Here's how the part is built. I have some questions about the finished solid (model axes, mm). A direction names the side the tool comes from. Coordinates: 2 decimals unless noted, no trailing zeros. Write each loop counter-clockwise with the first axis right and the second up, starting at its lowest first coordinate (ties: lowest second). Pieces come first, ordered by that corner, then holes. Notation, with made-up numbers: (-3.75, -27) -> (11.25, -27) arc R20 cw to (11.25, -20) -> close; hole circle Ø7 at (27.5, 74.25). An arc over 180 degrees is marked (long way). Put each result on its own line as item: value. Start each with the question number.
Item 1: On a 3-axis mill with a long thin cutter (end or side, diameter ignored), from which of +Z, -Z, +X, -X, +Y, -Y can I reach the whole of each face in a straight line? I mean faces 1 (the face through (54.8, 2, -30)), 2 (the face through (9, 2, -42.5)), 3 (the face through (-56.5, 1.48, -41.07)). Say none if no direction works.
Item 2: I want a section at B-B, the plane z = 9. List the corners of the cut face in (x, y) for me, then the cut area to 3 significant figures.
Item 3: For pin 1 (0.9 mm diameter, centred on y = 1, z = -33, fed in from +X); pin 2 (1.5 mm diameter, centred on x = -41.5, y = 1.5, fed in from -Z), each with a flat end and sliding along its axis, tell me the tip position at first contact or that it passes through.
Item 4: I want a section at C-C, the plane x = -98. List the corners of the cut face in (y, z) for me, then the cut area to 3 significant figures.
Item 5: If we mould it in two halves opening along X, with no side actions, what happens to faces 4 (the face through (-93.982, 1.521, -1.905)), 5 (the face through (-45, 1, -22.5)), 6 (the face through (73.5, 1.52, -21.07))? For each: released by +X, released by -X, zero draft, split by the parting line, or undercut.
Item 6: I want a section at A-A, the plane y = 0.5. List the corners of the cut face in (x, z) for me, then the cut area to 3 significant figures.
Item 7: I need wall thicknesses on line 1 (X direction, y = 1.05, z = -28); line 2 (X direction, y = 2.2, z = -25); line 3 (X direction, y = 2.15, z = -4). Which ranges of each line are inside material? Lowest first, please. Write a range as [from, to].
from build123d import *

# Parameters (mm, degrees)
SKETCH1_W           = 150
SKETCH1_H           = 45
BOSS_EXTRUDE1_DEPTH = 3
FILLET1_R           = 30
SKETCH2_W           = 89.6
SKETCH2_H           = 20
BOSS_EXTRUDE2_DEPTH = 3
FILLET2_R           = 30
SKETCH3_R           = 0.8
SKETCH3_R_2         = 0.899402105
CUT_EXTRUDE1_DEPTH  = 118.962917902
FILLET3_R           = 5


with BuildPart() as part:
    # Sketch1 → Boss-Extrude1 (new body)
    with BuildSketch(Plane(origin=(0, 0, 0), x_dir=(1, 0, 0), z_dir=(0, 1, 0))):
        Rectangle(SKETCH1_W, SKETCH1_H)
    extrude(amount=BOSS_EXTRUDE1_DEPTH)

    # Fillet1
    fillet1_edges = [part.edges().sort_by_distance(p)[0] for p in [
        (75, 1.5, 22.5),
    ]]
    fillet(fillet1_edges, radius=FILLET1_R)

    # Sketch2 → Boss-Extrude2 (add)
    with BuildSketch(Plane(origin=(0, 3, 0), x_dir=(1, 0, 0), z_dir=(0, 1, 0))):
        Polygon((-75, 22.5), (-55, 22.5), (-55, 42.5), (-110, 42.5), (-110, 22.5), align=None)
        Polygon((-75, -22.5), (-75, 22.5), (-110, 22.5), align=None)
        with Locations((10, 32.5)):
            Rectangle(SKETCH2_W, SKETCH2_H)
    extrude(amount=-BOSS_EXTRUDE2_DEPTH)

    # Fillet2
    fillet2_edges = [part.edges().sort_by_distance(p)[0] for p in [
        (-110, 1.5, -22.5),
        (-75, 1.5, 22.5),
    ]]
    fillet(fillet2_edges, radius=FILLET2_R)

    # Sketch3 → Cut-Extrude1 (cut, through all)
    with BuildSketch(Plane(origin=(0, 3, 0), x_dir=(1, 0, 0), z_dir=(0, 1, 0))):
        with Locations((-55, 22.5)):
            Circle(SKETCH3_R)
        with Locations((-34.8, 22.5)):
            Circle(SKETCH3_R)
        with Locations((54.8, 22.5)):
            Circle(SKETCH3_R_2)
    extrude(amount=-CUT_EXTRUDE1_DEPTH, mode=Mode.SUBTRACT)

    # Fillet3
    fillet3_edges = [part.edges().sort_by_distance(p)[0] for p in [
        (-55, 1.5, -42.5),
        (-110, 1.5, -42.5),
        (-34.8, 1.5, -42.5),
        (54.8, 1.5, -42.5),
        (75, 1.5, -22.5),
    ]]
    fillet(fillet3_edges, radius=FILLET3_R)


solid = part.part
Calculated:
1. face 1: -Z, +X, +Y, -Y
1. face 2: -Z, +X, -X, +Y, -Y
1. face 3: -Z, +Y, -Y
2. outline: (-85.5, 0) -> (70.05, 0) -> (70.05, 3) -> (-85.5, 3) -> close
2. area: 467 mm2
3. pin 1: stops at x = 54.8
3. pin 2: stops at z = -22.5
4. outline: (0, -42.5) -> (3, -42.5) -> (3, -7.07) -> (0, -7.07) -> close
4. area: 106 mm2
5. face 4: released by -X
5. face 5: undercut
5. face 6: released by +X
6. outline: (-110, -37.5) arc R5 ccw to (-105, -42.5) -> (-60, -42.5) arc R5 ccw to (-55, -37.5) -> (-55, -23.3) arc R0.8 cw (long way) to (-54.2, -22.5) -> (-35.6, -22.5) arc R0.8 cw (long way) to (-34.8, -23.3) -> (-34.8, -37.5) arc R5 ccw to (-29.8, -42.5) -> (49.8, -42.5) arc R5 ccw to (54.8, -37.5) -> (54.8, -23.4) arc R0.9 cw (long way) to (55.7, -22.5) -> (70, -22.5) arc R5 ccw to (75, -17.5) -> (75, -7.5) arc R30 ccw to (45, 22.5) -> (-60.33, 22.5) arc R30 ccw to (-84.01, 10.92) -> (-103.68, -14.38) arc R30 ccw to (-110, -32.79) -> close
6. area: 10,200 mm2
7. line 1: x = [-109.61, -55], [-34.8, 54.8]
7. line 2: x = [-108.97, -55], [-34.8, 54.8]
7. line 3: x = [-95.61, 74.8]
